```python
from build123d import *

# Parameters (mm, degrees)
F0_R     = 2
F0_R_2   = 3
F1_DEPTH = 20
F2_R     = 3.99999


# Not quite as in the source:
# - a fillet or chamfer is up to 0.001 mm smaller than in the source, because OpenCascade refuses the exact size


with BuildPart() as f1:
    # F0 (on Top) → F1 (new body)
    with BuildSketch(Plane.XY):
        with BuildLine():
            Line((-32.5, 60), (-55, 60))
            ThreePointArc((-55, 60), (-58.5355339059, 58.5355339059), (-60, 55))
            Line((-60, 55), (-60, 32.5))
            Line((-60, 32.5), (-68, 32.5))
            Line((-68, 32.5), (-68, -32.5))
            Line((-68, -32.5), (-60, -32.5))
            Line((-60, -32.5), (-60, -50))
            ThreePointArc((-60, -50), (-57.0710678119, -57.0710678119), (-50, -60))
            Line((-50, -60), (-32.5, -60))
            Line((-32.5, -60), (-32.5, -68))
            Line((-32.5, -68), (32.5, -68))
            Line((32.5, -68), (32.5, -60))
            Line((32.5, -60), (45, -60))
            ThreePointArc((45, -60), (55.6066017178, -55.6066017178), (60, -45))
            Line((60, -45), (60, -32.5))
            Line((60, -32.5), (68, -32.5))
            Line((68, -32.5), (68, 32.5))
            Line((68, 32.5), (60, 32.5))
            Line((60, 32.5), (60, 40))
            ThreePointArc((60, 40), (54.1421356237, 54.1421356237), (40, 60))
            Line((40, 60), (32.5, 60))
            Line((32.5, 60), (32.5, 68))
            Line((32.5, 68), (-32.5, 68))
            Line((-32.5, 68), (-32.5, 60))
        make_face()
        with Locations((-50, -50)):
            Circle(F0_R, mode=Mode.SUBTRACT)
        with Locations((-27.5, -63)):
            Circle(F0_R_2, mode=Mode.SUBTRACT)
        with Locations((-63, -27.5)):
            Circle(F0_R_2, mode=Mode.SUBTRACT)
        with Locations((27.5, -63)):
            Circle(F0_R_2, mode=Mode.SUBTRACT)
        with Locations((45, -45)):
            Circle(F0_R, mode=Mode.SUBTRACT)
        with Locations((63, -27.5)):
            Circle(F0_R_2, mode=Mode.SUBTRACT)
        with Locations((-63, 27.5)):
            Circle(F0_R_2, mode=Mode.SUBTRACT)
        with Locations((-55, 55)):
            Circle(F0_R, mode=Mode.SUBTRACT)
        with Locations((-27.5, 63)):
            Circle(F0_R_2, mode=Mode.SUBTRACT)
        with Locations((63, 27.5)):
            Circle(F0_R_2, mode=Mode.SUBTRACT)
        with Locations((27.5, 63)):
            Circle(F0_R_2, mode=Mode.SUBTRACT)
        with Locations((40, 40)):
            Circle(F0_R, mode=Mode.SUBTRACT)
    extrude(amount=F1_DEPTH)

    # F2 (radius 4 in the source; OpenCascade refuses exactly that, so slightly less here)
    f2_edges = [f1.edges().sort_by_distance(p)[0] for p in [
        (-60, 32.5, 10),
        (-68, 32.5, 10),
        (-32.5, 60, 10),
        (-32.5, 68, 10),
        (32.5, 68, 10),
        (-68, -32.5, 10),
        (-32.5, -68, 10),
        (60, -32.5, 10),
        (68, -32.5, 10),
        (68, 32.5, 10),
        (32.5, -60, 10),
        (32.5, -68, 10),
        (-60, -32.5, 10),
        (-32.5, -60, 10),
        (60, 32.5, 10),
        (32.5, 60, 10),
    ]]
    fillet(f2_edges, radius=F2_R)


solid = f1.part
```
Verification items for the finished model (mm, model axes). A direction names the side the tool comes from. Coordinates: 2 decimals unless noted, no trailing zeros. Loops run counter-clockwise (first coordinate to the right, second up) from the corner with the lowest first, then second, coordinate; pieces in that order, holes last. Notation, with made-up numbers: (-6.75, -5.75) - (5.25, -5.75) arc R31 cw to (5.25, 21.25) - close; hole circle Ø10 at (-17.75, 67.5). An arc over 180 degrees is marked (long way). Answer as a JSON object with one key per item and string values.
(1) Mould release check, pull along X, two halves, no side actions. Record for faces 4 (the cylindrical face through (-31.359, 66.797, 10.14)), 5 (the flat face through (0, -68, 10)), 6 (the cylindrical face through (25.29, -60.97, 9.86)): pulls with the +X half, pulls with the -X half, needs draft (parallel to the pull), parting line crosses it, or undercut.
Response:
{"face 4": "pulls with the -X half", "face 5": "needs draft", "face 6": "undercut"}
(2) Cross-section at A-A, the plane x = -26.5. Record the boundary of the cut face in (y, z).
Response:
{"outline": "(-68, 0) - (-65.83, 0) - (-65.83, 20) - (-68, 20) - close; (-60.17, 0) - (60.17, 0) - (60.17, 20) - (-60.17, 20) - close; (65.83, 0) - (68, 0) - (68, 20) - (65.83, 20) - close"}
(3) Cross-section at C-C, the plane x = 57.5. Record the boundary of the cut face in (y, z), then the cut area to 3 significant figures.
Response:
{"outline": "(-53.29, 0) - (49.68, 0) - (49.68, 20) - (-53.29, 20) - close", "area": "2,060 mm²"}
(4) Cross-section at B-B, the plane z = 12.5. Count the separate pieces of the cut face and the enclosed holes in it, then the cut area to 3 significant figures.
Response:
{"separate pieces": "1", "enclosed holes": "12", "area": "16,000 mm²"}
(5) Go/stop test with flat-tipped pins: pin 1 Ø2.5 at (x, z) = (39, 8) entering from -Y; pin 2 Ø3.5 at (x, y) = (63, -27.5) entering from +Z; pin 3 Ø4.5 at (y, z) = (-41.5, 7) entering from +X; pin 4 Ø6 at (x, z) = (42.5, 15) entering from +Y. Record where each tip stops, or that it passes through.
Response:
{"pin 1": "stops at y = -60", "pin 2": "passes through", "pin 3": "stops at x = 60", "pin 4": "stops at y = 60"}
(6) Access from +Z, -Z, +X, -X, +Y, -Y to the whole of each face (thin tool, end or side, straight path). Record for faces 1 (the cylindrical face through (-61.203, -33.641, 10.14)), 2 (the flat face through (60, 38, 10)), 3 (the flat face through (-60, 46, 10)).
Response:
{"face 1": "+Z, -Z, -X, -Y", "face 2": "+Z, -Z, +X, +Y", "face 3": "+Z, -Z, -X, +Y"}
(7) Scan lines: line 1 along Y through (x, z) = (27.5, 15.25); line 2 along Y through (x, z) = (63, 9.5); line 3 along Y through (x, z) = (40, 7.25). Record each from-to range of solid material in increasing order.
Response:
{"line 1": "y = -68 to -66, -60 to 60, 66 to 68", "line 2": "y = -32.63 to -30.5, -24.5 to 24.5, 30.5 to 32.63", "line 3": "y = -60 to 38, 42 to 60"}
